For this review, take the finished solid that the model builds, in its own axes (mm). Round coordinates to 2 decimals unless told otherwise and drop trailing zeros. Loops run counter-clockwise (first coordinate to the right, second up) from the corner with the lowest first, then second, coordinate; pieces in that order, holes last.
1. Consider section A-A on z = 2.4. State the section outline as (x, y) points, then the cut area to 3 significant figures.
2. Consider section D-D on y = 84.5. State the section outline as (x, z) points, then the cut area to 3 significant figures.
3. To check wall thickness, follow line 1 along X through (y, z) = (67.5, 0.45); line 2 along Y through (x, z) = (0, 2.45); line 3 along X through (y, z) = (30, 1.95). State the ranges of each line that lie inside material, in increasing order.
4. Consider section C-C on x = 0. State the section outline as (y, z) points.
5. Clearance check with a flat-ended pin moving along its axis: pin 1 Ø1.5 at (x, z) = (-1, 1.5) entering from +Y. State where the tip first meets the part, or that it passes through.
6. Consider section B-B on y = 30. State the section outline as (x, z) points.
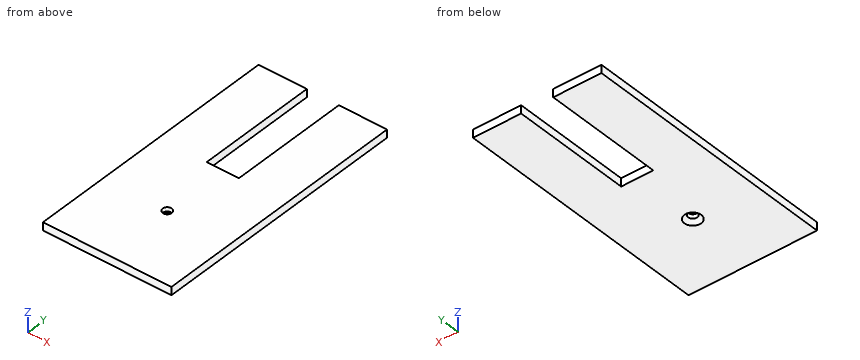
Autodesk Inventor part; units mm, degrees
ref_plane "Plan YZ" through (0, 0, 0) normal (1, 0, 0) x (0, 1, 0)
ref_plane "Plan XZ" through (0, 0, 0) normal (0, 1, 0) x (-1, 0, 0)
ref_plane "Plan XY" through (0, 0, 0) normal (0, 0, 1) x (1, 0, 0)
sketch "Esquisse6" plane through (0, 0, 0) normal (0, 0, 1) x (1, 0, 0)
  line L0 (0, -20) -> (0, 120) construction
  line L1 (-24, 0) -> (24, 0)
  line L2 (24, 0) -> (24, 100)
  line L3 (24, 100) -> (6, 100)
  line L4 (6, 100) -> (6, 55)
  line L5 (6, 55) -> (-6, 55)
  line L6 (-6, 55) -> (-6, 100)
  line L7 (-6, 100) -> (-24, 100)
  line L8 (-24, 100) -> (-24, 0)
  line L9 (-33.6, 0) -> (33.6, 0) construction
  point P0 (0, 0)
  dimension "d0" = 100
  dimension "d1" = 48
  dimension "d2" = 12
  dimension "d3" = 45
extrude "Extrusion1" add sketch "Esquisse6" along normal blind 3
sketch "Esquisse7" plane through (0, 0, 0) normal (0, 0, -1) x (-1, 0, 0)
  line L0 (0, -20) -> (0, 120) construction
  line L1 (-24, 0) -> (24, 0)
  point P0 (0, 0)
  point P1 (0, 30)
  dimension "d24" = 30
sketch "Esquisse8" plane through (0, 0, 3) normal (0, 0, 1) x (1, 0, 0)
  line L0 (24, 100) -> (24, 0)
  line L1 (-24, 0) -> (24, 0)
  line L2 (24, 0) -> (24, 3)
  line L3 (24, 3) -> (-24, 3)
  line L4 (-24, 3) -> (-24, 0)
  line L5 (-24, 100) -> (-24, 0)
  line L6 (24, 0) -> (24, 100)
  line L7 (-24, 0) -> (24, 0)
  point P0 (0, 0)
  dimension "d21" = 3
extrude "Extrusion3" cut sketch "Esquisse8" against normal through all
hole "Perçage1" at (0, 30, 0) direction (0, 0, 1) diameter 3.4 end through all countersink diameter 6.3 countersink angle 90
properties part number "S1702_replat" material "Plastique PMMA"
Resolved:
1. outline: (-24, 3) - (24, 3) - (24, 100) - (6, 100) - (6, 55) - (-6, 55) - (-6, 100) - (-24, 100) - close; hole circle Ø3.4 at (0, 30)
1. area: 4,110 mm2
2. outline: (-24, 0) - (-6, 0) - (-6, 3) - (-24, 3) - close; (6, 0) - (24, 0) - (24, 3) - (6, 3) - close
2. area: 108 mm2
3. line 1: x = -24 to -6, 6 to 24
3. line 2: y = 3 to 28.3, 31.7 to 55
3. line 3: x = -24 to -1.7, 1.7 to 24
4. outline: (3, 0) - (26.85, 0) - (28.3, 1.45) - (28.3, 3) - (3, 3) - close; (31.7, 1.45) - (33.15, 0) - (55, 0) - (55, 3) - (31.7, 3) - close
5. pin 1: stops at y = 55
6. outline: (-24, 0) - (-3.15, 0) - (-1.7, 1.45) - (-1.7, 3) - (-24, 3) - close; (1.7, 1.45) - (3.15, 0) - (24, 0) - (24, 3) - (1.7, 3) - close
